Source: CAD feature listing. Evaluate the final solid. Frame: model axes, mm. Round coordinates to 2 decimals unless told otherwise and drop trailing zeros. Write each loop counter-clockwise with the first axis right and the second up, starting at its lowest first coordinate (ties: lowest second). Pieces come first, ordered by that corner, then holes. Notation, with made-up numbers: M 69,-35.5 L 82,-35.5 A27 cw 82,-19.5 Z; hole C 12.25,41.5 d9. An arc over 180 degrees is marked long. Use a Markdown table: item, result.
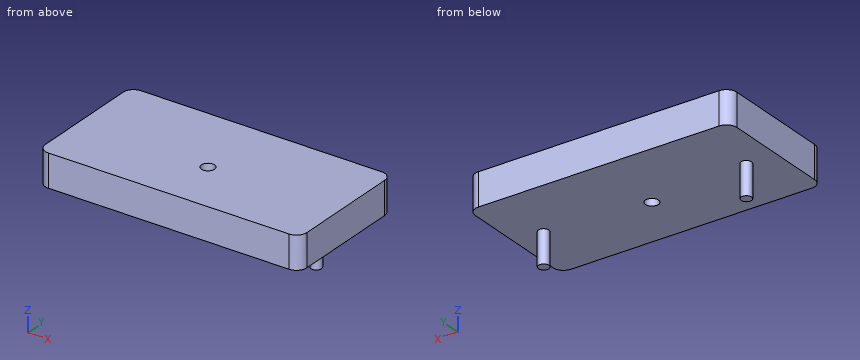
Autodesk Inventor part; units mm, degrees
ref_plane "YZ Plane" through (0, 0, 0) normal (1, 0, 0) x (0, 1, 0)
ref_plane "XZ Plane" through (0, 0, 0) normal (0, 1, 0) x (-1, 0, 0)
ref_plane "XY Plane" through (0, 0, 0) normal (0, 0, 1) x (1, 0, 0)
sketch "Sketch1" plane through (0, 0, 0) normal (0, 0, 1) x (1, 0, 0)
  line L0 (-100, 50) -> (100, 50)
  line L1 (100, 50) -> (100, -50)
  line L2 (100, -50) -> (-100, -50)
  line L3 (-100, -50) -> (-100, 50)
  line L4 (-100, 50) -> (100, -50) construction
  line L5 (100, 50) -> (-100, -50) construction
  point P0 (0, 0)
  dimension "d0" = 200
  dimension "d1" = 100
extrude "Extrusion1" add sketch "Sketch1" along normal mid plane 25
fillet "Fillet1" radius 8 4 edges at (100, 50, 0) (-100, 50, 0) (100, -50, 0) (-100, -50, 0)
sketch "Sketch2" plane through (0, 0, -12.5) normal (0, 0, -1) x (-1, 0, 0)
  line L0 (-77.5, 10) -> (77.5, 10)
  line L1 (77.5, 10) -> (77.5, -10)
  line L2 (77.5, -10) -> (-77.5, -10)
  line L3 (-77.5, -10) -> (-77.5, 10)
  line L4 (-77.5, 10) -> (77.5, -10) construction
  line L5 (77.5, 10) -> (-77.5, -10) construction
  circle A0 centre (-77.5, 0) radius 4
  circle A1 centre (77.5, 0) radius 4
  point P0 (0, 0)
  dimension "d5" = 155
  dimension "d6" = 20
  dimension "d7" = 8
  dimension "d8" = 8
extrude "Extrusion2" add sketch "Sketch2" along normal blind 25 contours A0 L3 | L3 A0 | A1 L1 | L1 A1
sketch "Sketch3" plane through (0, 0, -12.5) normal (0, 0, -1) x (-1, 0, 0)
  line L0 (-92, -50) -> (92, -50)
  line L1 (0, -50) -> (0, -7.5)
  circle A0 centre (0, -7.5) radius 5
  point P0 (0, 0)
  dimension "d11" = 42.5
  dimension "d12" = 10
extrude "Extrusion3" cut sketch "Sketch3" against normal blind 25
properties part number "CAJA REDUCTORA"
Q1. Line query: L1, parallel to Y at x = 0, z = -5; L2, parallel to X at y = -7.5, z = 0.5; L3, parallel to Z at x = -65, y = 4. Output: solid intervals per line, ascending.
Results are:
| item | result |
|---|---|
| L1 | -50 to -12.5, -2.5 to 50 |
| L2 | -100 to -5, 5 to 100 |
| L3 | -12.5 to 12.5 |
Q2. Section B-B on y = -7.5. Return loops of the section in (x, z).
Results are:
| item | result |
|---|---|
| outline | M -100,-12.5 L -5,-12.5 L -5,12.5 L -100,12.5 Z; M 5,-12.5 L 100,-12.5 L 100,12.5 L 5,12.5 Z |
Q3. Section A-A on x = 0. Return loops of the section in (y, z), plus the area to 3 significant figures.
Results are:
| item | result |
|---|---|
| outline | M -50,-12.5 L -12.5,-12.5 L -12.5,12.5 L -50,12.5 Z; M -2.5,-12.5 L 50,-12.5 L 50,12.5 L -2.5,12.5 Z |
| area | 2,250 mm^2 |
Q4. First-contact query: pin 1 Ø8 at (x, y) = (71, -26) entering from -Z; pin 2 Ø6 at (x, y) = (0, -7.5) entering from +Z. Flat tips, straight axial feed; report the tip coordinate or a pass-through.
Results are:
| item | result |
|---|---|
| pin 1 | z = -12.5 |
| pin 2 | through |
Q5. Section C-C on x = 77.5. Return loops of the section in (y, z).
Results are:
| item | result |
|---|---|
| outline | M -50,-12.5 L -4,-12.5 L -4,-37.5 L 4,-37.5 L 4,-12.5 L 50,-12.5 L 50,12.5 L -50,12.5 Z |
Q6. Section D-D on z = -31. Return loops of the section in (x, y).
Results are:
| item | result |
|---|---|
| outline | C -77.5,0 d8; C 77.5,0 d8 |
